from build123d import *

# Parameters (mm, degrees)
F4_DEPTH  = 40
F5_DEPTH  = 10
F6_DEPTH  = 10
F7_R      = 10
F8_R      = 2.5
F10_DEPTH = 100.001
F9_R      = 2.5
F11_DEPTH = 85.001
F12_DEPTH = 5
F13_DEPTH = 3
F0_R      = 10
F0_R_2    = 7.5
F14_DEPTH = 10
F15_R     = 10
F15_R_2   = 7.5
F16_DEPTH = 5
F19_D     = 4.2
F19_DEPTH = 10
F19_TIP   = 1.2618073


with BuildPart() as f4:
    # F0 (on Front) → F4 (new body)
    with BuildSketch(Plane.XZ):
        with BuildLine():
            Line((0, -50), (0, -85))
            Line((0, -85), (5, -85))
            Line((5, -85), (5, -7))
            ThreePointArc((5, -7), (5.5857864376, -5.5857864376), (7, -5))
            Line((7, -5), (100, -5))
            Line((100, -5), (100, 0))
            Line((100, 0), (50, 0))
            Line((50, 0), (7, 0))
            ThreePointArc((7, 0), (2.0502525317, -2.0502525317), (0, -7))
            Line((0, -7), (0, -50))
        make_face()
    extrude(amount=F4_DEPTH)

    # F2 (on Right) → F5 (cut)
    with BuildSketch(Plane.YZ):
        Polygon((-20, -26.1649281481), (-20, 0), (-40, 0), (-40, -85), (-32.5, -85), (-32.5, -41.0618480555), align=None)
    extrude(amount=F5_DEPTH, mode=Mode.SUBTRACT)

    # F3 (on Top) → F6 (cut)
    with BuildSketch(Plane.XY):
        Polygon((30.2180073765, -20), (0, -20), (0, -40), (47, -40), align=None)
    extrude(amount=-F6_DEPTH, mode=Mode.SUBTRACT)

    # F7
    f7_edges = [f4.edges().sort_by_distance(p)[0] for p in [
        (2.5, -32.5, -85),
        (100, -40, -2.5),
    ]]
    fillet(f7_edges, radius=F7_R)

    # F8 (on Right) → F10 (cut, through all)
    with BuildSketch(Plane.YZ):
        with Locations((-17.5, -70)):
            Circle(F8_R)
        with Locations((-17.5, -45)):
            Circle(F8_R)
    extrude(amount=F10_DEPTH, mode=Mode.SUBTRACT)

    # F9 (on Top) → F11 (cut, through all)
    with BuildSketch(Plane.XY):
        with Locations((50, -20)):
            Circle(F9_R)
        with Locations((80, -20)):
            Circle(F9_R)
    extrude(amount=-F11_DEPTH, mode=Mode.SUBTRACT)

    # F0 (on Front) → F12 (join)
    with BuildSketch(Plane.XZ):
        with BuildLine():
            Line((-27.5303153895, 7.5246185085), (0, -50))
            Line((0, -50), (0, -7))
            ThreePointArc((0, -7), (2.0502525317, -2.0502525317), (7, 0))
            Line((7, 0), (50, 0))
            Line((50, 0), (-7.5246185085, 27.5303153895))
            ThreePointArc((-7.5246185085, 27.5303153895), (-1.3088471294, 21.9959138824), (1, 14))
            ThreePointArc((1, 14), (-10.6799646721, -0.6279651839), (-27.5303153895, 7.5246185085))
        make_face()
        with BuildLine():
            Line((-3, -36.782099822), (-19.0324950336, -3.2821871804))
            ThreePointArc((-19.0324950336, -3.2821871804), (-10.6526660041, -3.686021461), (-3, -0.2478068488))
            Line((-3, -0.2478068488), (-3, -36.782099822))
        make_face(mode=Mode.SUBTRACT)
        with BuildLine():
            ThreePointArc((0.2478068488, 3), (3.686021461, 10.6526660041), (3.2821871804, 19.0324950336))
            Line((3.2821871804, 19.0324950336), (36.782099822, 3))
            Line((36.782099822, 3), (0.2478068488, 3))
        make_face(mode=Mode.SUBTRACT)
    extrude(amount=F12_DEPTH)

    # F0 (on Front) → F13 (join)
    with BuildSketch(Plane.XZ):
        with BuildLine():
            Line((36.782099822, 3), (3.2821871804, 19.0324950336))
            ThreePointArc((3.2821871804, 19.0324950336), (3.686021461, 10.6526660041), (0.2478068488, 3))
            Line((0.2478068488, 3), (36.782099822, 3))
        make_face()
        with BuildLine():
            ThreePointArc((-3, -0.2478068488), (-10.6526660041, -3.686021461), (-19.0324950336, -3.2821871804))
            Line((-19.0324950336, -3.2821871804), (-3, -36.782099822))
            Line((-3, -36.782099822), (-3, -0.2478068488))
        make_face()
    extrude(amount=F13_DEPTH)

    # F0 (on Front) → F14 (join)
    with BuildSketch(Plane.XZ):
        with BuildLine():
            ThreePointArc((-7.5246185085, 27.5303153895), (-24.6066017178, 24.6066017178), (-27.5303153895, 7.5246185085))
            ThreePointArc((-27.5303153895, 7.5246185085), (-10.6799646721, -0.6279651839), (1, 14))
            ThreePointArc((1, 14), (-1.3088471294, 21.9959138824), (-7.5246185085, 27.5303153895))
        make_face()
        with Locations((-14, 14)):
            Circle(F0_R, mode=Mode.SUBTRACT)
        with Locations((-14, 14)):
            Circle(F0_R)
        with Locations((-14, 14)):
            Circle(F0_R_2, mode=Mode.SUBTRACT)
    extrude(amount=F14_DEPTH)

    # F15 (on face) → F16 (cut)
    with BuildSketch(Plane.XZ.offset(10)):
        with Locations((-14, 14)):
            Circle(F15_R)
        with Locations((-14, 14)):
            Circle(F15_R_2, mode=Mode.SUBTRACT)
    extrude(amount=-F16_DEPTH, mode=Mode.SUBTRACT)

    # F17: F4 across plane


with BuildPart() as f4_1:
    add(f4.part)
    add(f4.part.mirror(Plane.XZ))

    # F19
    with Locations(Plane(origin=(-24.6066017178, 0, 24.6066017178), x_dir=(0, -1, 0), z_dir=(-0.7071067812, 0, 0.7071067812))):
        with Locations((0, 0)):
            Hole(F19_D / 2, depth=F19_DEPTH)
            with Locations((0, 0, -(F19_DEPTH + F19_TIP / 2))):  # 118° drill point
                Cone(0, F19_D / 2, F19_TIP, mode=Mode.SUBTRACT)


solid = f4_1.part
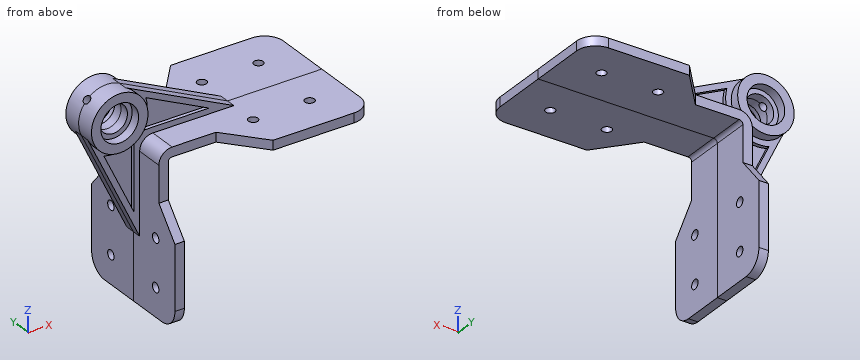
Model file for the job. Use its own axes, mm. Give positions to 0.01 mm unless a question says otherwise; leave off trailing zeros. Order: outer loops, then holes, each group sorted by start corner. A loop starts at its lowest first (then second) coordinate and runs counter-clockwise, first axis right, second up. Notation, with made-up numbers: (6, 59) -> (17, 59) arc R22 ccw to (17, 95) -> close; hole circle Ø2 at (58, -15.75). An arc over 180 degrees is marked (long way). Use CSV: the item, a comma, the result in double quotes.
1. Band-saw the part on D-D, the plane x = 69. Give the cut face in (y, z), then the cut area to 3 significant figures.
Outcome:
outline,"(-40, -5) -> (40, -5) -> (40, 0) -> (-40, 0) -> close"
area,"400 mm²"
2. Drop flat-ended pins along their axis: pin 1 (4.5 mm diameter, centred on x = 50, y = 20, fed in from +Z); pin 2 (8 mm diameter, centred on x = 0.5, z = -60.5, fed in from +Y); pin 3 (8 mm diameter, centred on x = 80, y = 20, fed in from +Z); pin 4 (22 mm diameter, centred on x = -18.5, z = 12.5, fed in from +Y). Give the stop position or say it passes through.
Outcome:
pin 1,"through"
pin 2,"y = 32.5"
pin 3,"z = 0"
pin 4,"y = 10"
3. Drill centre lines: line 1 along Y through (x, z) = (4, -70); line 2 along Z through (x, y) = (2, -17); line 3 along Z through (x, y) = (3.3, -17.5). Where is each one in solid material? Low to high. Write a range as from..to.
Outcome:
line 1,"-32.5..-20, -15..15, 20..32.5"
line 2,"-85..-72.45, -67.55..-47.45, -42.55..-2.1"
line 3,"-85..-72.5, -67.5..-47.5, -42.5..-1.06"
4. Band-saw the part on A-A, the plane z = -45. Give the cut face in (x, y).
Outcome:
outline,"(-2.39, -5) -> (0, -5) -> (0, -15) -> (5, -15) -> (5, 15) -> (0, 15) -> (0, 5) -> (-2.39, 5) -> close; (0, -32.5) -> (5, -32.5) -> (5, -20) -> (0, -20) -> close; (0, 20) -> (5, 20) -> (5, 32.5) -> (0, 32.5) -> close"
5. Band-saw the part on B-B, the plane y = 27. Give the cut face in (x, z), then the cut area to 3 significant figures.
Outcome:
outline,"(0, -83.93) -> (5, -83.93) -> (5, -34.51) -> (0, -34.51) -> close; (36.09, -5) -> (100, -5) -> (100, 0) -> (36.09, 0) -> close"
area,"567 mm²"
6. Band-saw the part on C-C, the plane z = 14. Give the cut face in (x, y), then the cut area to 3 significant figures.
Outcome:
outline,"(-29, -10) -> (-24, -10) -> (-24, -5) -> (-21.5, -5) -> (-21.5, 5) -> (-24, 5) -> (-24, 10) -> (-29, 10) -> close; (-6.5, -5) -> (-4, -5) -> (-4, -10) -> (1, -10) -> (1, -5) -> (4, -5) -> (4, -3) -> (13.8, -3) -> (13.8, -5) -> (20.75, -5) -> (20.75, 5) -> (13.8, 5) -> (13.8, 3) -> (4, 3) -> (4, 5) -> (1, 5) -> (1, 10) -> (-4, 10) -> (-4, 5) -> (-6.5, 5) -> close"
area,"408 mm²"
